Autodesk Fusion 360 part; units mm, degrees
sketch "Sketch1" plane through (0, 0, 0) normal (0, 0, 1) x (1, 0, 0) in component "Component"
  line L0 (-4.9635, 8.6391) -> (5.0365, 8.6391)
  line L1 (-9.9634, 0.021) -> (-4.9634, 8.6813)
  line L2 (-4.9999, -8.6181) -> (-9.9999, 0.0422)
  line L3 (4.9635, -8.6391) -> (-5.0365, -8.6391)
  line L4 (9.9634, -0.021) -> (4.9634, -8.6813)
  line L5 (4.9999, 8.6181) -> (9.9999, -0.0422)
  dimension "d2" = 10
  dimension "d4" = 360
  dimension "d5" = 10
  dimension "d6" = 10
sketch "Sketch2" plane through (0, 0, 0) normal (0, 0, 1) x (1, 0, 0) in component "Component"
  line L0 (23.094, 40) -> (0, 0) construction
  line L1 (0, 0) -> (-23.094, 40) construction
  line L2 (1.925, 38) -> (1.925, 30)
  line L3 (1.925, 30) -> (-1.925, 30)
  line L4 (-1.925, 30) -> (-1.925, 38)
  line L5 (-23.094, 40) -> (-3.925, 40)
  line L6 (3.925, 40) -> (23.094, 40)
  line L7 (-3.925, 40) -> (-1.925, 38)
  line L8 (0, 30) -> (0, 40) construction
  line L9 (3.925, 40) -> (1.925, 38)
  line L10 (-32.6785, 23.3991) -> (-23.094, 40)
  line L11 (-32.6785, 23.3991) -> (-31.9465, 20.6671)
  line L12 (-26.9433, 13.3329) -> (-33.8715, 17.3329)
  line L13 (-25.9808, 15) -> (-34.641, 20) construction
  line L14 (-36.6035, 16.6009) -> (-33.8715, 17.3329)
  line L15 (-46.188, 0) -> (-36.6035, 16.6009)
  line L16 (-25.0183, 16.6671) -> (-26.9433, 13.3329)
  line L17 (-31.9465, 20.6671) -> (-25.0183, 16.6671)
  line L18 (-36.6035, -16.6009) -> (-46.188, 0)
  line L19 (-36.6035, -16.6009) -> (-33.8715, -17.3329)
  line L20 (-25.0183, -16.6671) -> (-31.9465, -20.6671)
  line L21 (-25.9808, -15) -> (-34.641, -20) construction
  line L22 (-32.6785, -23.3991) -> (-31.9465, -20.6671)
  line L23 (-23.094, -40) -> (-32.6785, -23.3991)
  line L24 (-26.9433, -13.3329) -> (-25.0183, -16.6671)
  line L25 (-33.8715, -17.3329) -> (-26.9433, -13.3329)
  line L26 (-3.925, -40) -> (-23.094, -40)
  line L27 (-3.925, -40) -> (-1.925, -38)
  line L28 (1.925, -30) -> (1.925, -38)
  line L29 (0, -30) -> (0, -40) construction
  line L30 (3.925, -40) -> (1.925, -38)
  line L31 (23.094, -40) -> (3.925, -40)
  line L32 (-1.925, -30) -> (1.925, -30)
  line L33 (-1.925, -38) -> (-1.925, -30)
  line L34 (32.6785, -23.3991) -> (23.094, -40)
  line L35 (32.6785, -23.3991) -> (31.9465, -20.6671)
  line L36 (26.9433, -13.3329) -> (33.8715, -17.3329)
  line L37 (25.9808, -15) -> (34.641, -20) construction
  line L38 (36.6035, -16.6009) -> (33.8715, -17.3329)
  line L39 (46.188, 0) -> (36.6035, -16.6009)
  line L40 (25.0183, -16.6671) -> (26.9433, -13.3329)
  line L41 (31.9465, -20.6671) -> (25.0183, -16.6671)
  line L42 (36.6035, 16.6009) -> (46.188, 0)
  line L43 (36.6035, 16.6009) -> (33.8715, 17.3329)
  line L44 (25.0183, 16.6671) -> (31.9465, 20.6671)
  line L45 (25.9808, 15) -> (34.641, 20) construction
  line L46 (32.6785, 23.3991) -> (31.9465, 20.6671)
  line L47 (23.094, 40) -> (32.6785, 23.3991)
  line L48 (26.9433, 13.3329) -> (25.0183, 16.6671)
  line L49 (33.8715, 17.3329) -> (26.9433, 13.3329)
  point P0 (0, 40)
  point P1 (0, 40)
  point P2 (-34.641, 20)
  point P3 (-34.641, 20)
  point P4 (-34.641, -20)
  point P5 (-34.641, -20)
  point P6 (0, -40)
  point P7 (0, -40)
  point P8 (34.641, -20)
  point P9 (34.641, -20)
  point P10 (34.641, 20)
  point P11 (34.641, 20)
  dimension "d8" = 40
  dimension "d10" = 60
  dimension "d22" = 45
  dimension "d23" = 2
  dimension "d24" = 3.85
  dimension "d25" = 10
  dimension "d27" = 360
extrude "Extrude1" add sketch "Sketch2" along normal blind 3
component "Component" placed x (1, 0, 0) y (0, 1, 0) z (0, 0, 1) at (0, 0, 0)
equation "Radius = 40 mm"
equation "d8 = Radius"
equation "d10 = Angle"
equation "Angle = ( 360 / NumberSides ) * 1 deg"
equation "Thickness = 4 mm"
equation "Kerf = 0.15 mm"
equation "Slot = 10 mm"
equation "Chamfer_Angle = 45 deg"
equation "Chamfer_Size = 2 mm"
equation "d22 = Chamfer_Angle"
equation "d23 = Chamfer_Size"
equation "d24 = Thickness - Kerf"
equation "d25 = Slot"
Read the model definition and answer for the solid it produces. Units are mm, in the model's axes. A direction names the side the tool comes from. Give positions to 0.01 mm unless a question says otherwise; leave off trailing zeros. Write each loop counter-clockwise with the first axis right and the second up, starting at its lowest first coordinate (ties: lowest second). Pieces come first, ordered by that corner, then holes. Notation, with made-up numbers: (-39.5, -16.5) -> (-13.5, -16.5) arc R11 cw to (-13.5, -4.5) -> close; hole circle Ø7 at (60.5, 55). An arc over 180 degrees is marked (long way). Answer as a JSON object with one key per item and string values. Group by question number.
1) A tool of negligible diameter and unlimited length cuts with its end or side. For faces 1 (the flat face through (-2.939, -39.014, 1.479)), 2 (the flat face through (-30.456, -15.361, 1.479)), 3 (the flat face through (32.318, 22.052, 1.479)), 4 (the flat face through (-32.318, -22.052, 1.479)), from which of +Z, -Z, +X, -X, +Y, -Y can it reach the whole face along a straight path? Write none if from no direction.
2) Consider L1, parallel to Y at x = 25.5, z = 2.4; L2, parallel to X at y = -15.5, z = 1.25; L3, parallel to X at y = -15, z = 2.45. Determine where each line is inside the solid, lowest interval first. Write a range as from..to.
3) Each of these flat-tipped pins is pushed along its axis until it touches: P1, Ø0.9, axis at y = 35, z = 1, coming from the +X side; P2, Ø1, axis at y = -9.5, z = 1, coming from the -X side; P3, Ø1.5, axis at y = 33, z = 2, coming from the -X side. Where does it stop, or does it pass through?
4) The mould has two halves that part along X. Classify faces 5 (the flat face through (-27.953, 31.583, 1.479)), 6 (the flat face through (-25.97, 15.02, 1.48)), 7 (the flat face through (-28.434, -18.639, 1.479)), 8 (the flat face through (41.329, 8.417, 1.479)): +X half, -X half, draft (parallel to the pull), parting line (faces both ways), or undercut.
5) Find section A-A (y = -4). Write down the section's boundary in (x, z), and give its area (3 significant figures).
6) Find section B-B (y = -25). Write down the section's boundary in (x, z), and give its area (3 significant figures).
Values follow:
{
 "1": {"face 1": "+Z, -Z, -Y", "face 2": "+Z, -Z", "face 3": "+Z, -Z, +X", "face 4": "+Z, -Z, -X"},
 "2": {"L1": "y = -35.83..-16.95, -15.83..15.83, 16.95..35.83", "L2": "x = -37.24..-30.7, -25.69..25.69, 30.7..37.24", "L3": "x = -37.53..-29.83, -25.98..25.98, 29.83..37.53"},
 "3": {"P1": "stops at x = 26.24", "P2": "stops at x = -40.99", "P3": "stops at x = -27.57"},
 "4": {"face 5": "-X half", "face 6": "undercut", "face 7": "undercut", "face 8": "+X half"},
 "5": {"outline": "(-43.88, 0) -> (43.88, 0) -> (43.88, 3) -> (-43.88, 3) -> close", "area": "263 mm2"},
 "6": {"outline": "(-31.75, 0) -> (31.75, 0) -> (31.75, 3) -> (-31.75, 3) -> close", "area": "191 mm2"}
}
